Source: CAD feature listing. Evaluate the final solid. Frame: model axes, mm. A direction names the side the tool comes from. Round coordinates to 2 decimals unless told otherwise and drop trailing zeros. Order: outer loops, then holes, each group sorted by start corner. A loop starts at its lowest first (then second) coordinate and runs counter-clockwise, first axis right, second up. Notation, with made-up numbers: M -33,-24.5 L -1,-24.5 A25 cw -1,-8.5 Z; hole C 50,83 d5. An arc over 180 degrees is marked long. Use CSV: the item, a comma, the result in double quotes. Start each with the question number.
```python
from build123d import *

# Parameters (mm, degrees)
F1_DEPTH = 25


with BuildPart() as f1:
    # F0 (on Front) → F1 (new body)
    with BuildSketch(Plane.XZ):
        with BuildLine():
            Line((0, 260), (0, 0))
            Line((0, 0), (2, 0))
            Line((2, 0), (2, 32.289786))
            Line((2, 32.289786), (227.065674, 257.35546))
            Line((227.065674, 257.35546), (268, 257.760407))
            Line((268, 257.760407), (268, 210))
            ThreePointArc((268, 210), (288, 190), (308, 210))
            Line((308, 210), (308, 260))
            Line((308, 260), (306, 260))
            Line((306, 260), (306, 210))
            ThreePointArc((306, 210), (288, 192), (270, 210))
            Line((270, 210), (270, 260))
            Line((270, 260), (0, 260))
        make_face()
        Polygon((2, 35.118214), (2, 255.128978), (224.208987, 257.3272), align=None, mode=Mode.SUBTRACT)
    extrude(amount=F1_DEPTH)


solid = f1.part
```
(1) Section D-D on x = 288. Return loops of the section in (y, z).
(2) Contact query for flat-ended pins moving along their axis: P1, Ø3, axis at x = 110, y = -21.5, coming from the -Z side; P2, Ø7.5, axis at y = -11.5, z = 189, coming from the +X side; P3, Ø5, axis at x = 226, y = -2.5, coming from the -Z side. Output: stop coordinate, or through.
(3) Draft query along Z for faces 1 (the face through (270, -12, 235)), 2 (the face through (137, -12, 260)), 3 (the face through (114.66, -12.32, 147.78)). Return one class per face: pulls with the +Z half, pulls with the -Z half, needs draft (parallel to the pull), parting line crosses it, or undercut.
(4) Section A-A on x = 199.5. Return loops of the section in (y, z), plus the area to 3 significant figures.
(5) Section C-C on y = -21.5. Return loops of the section in (x, z).
(6) Line query: line 1 along X through (y, z) = (-6.75, 213.5); line 2 along X through (y, z) = (-1.5, 241); line 3 along Z through (x, y) = (260.5, -5). Output: solid intervals per line, ascending.
(7) Reachability of faces 4 (the face through (306, -12, 235)), 5 (the face through (2, -12, 16)), 6 (the face through (112.96, -12.32, 143.25)), 7 (the face through (2, -12, 144)) from +Z, -Z, +X, -X, +Y, -Y: full face, straight path, thin tool, end or side. Return the list, or none.
(8) Section B-B on z = 42.5. Return loops of the section in (x, y), plus the area to 3 significant figures.
Results below:
1,outline,"M -25,190 L 0,190 L 0,192 L -25,192 Z"
2,P1,"stops at z = 138.79"
2,P2,"stops at x = 298.12"
2,P3,"stops at z = 253.79"
3,face 1,"needs draft"
3,face 2,"pulls with the +Z half"
3,face 3,"undercut"
4,outline,"M -25,229.79 L 0,229.79 L 0,232.62 L -25,232.62 Z; M -25,257.08 L 0,257.08 L 0,260 L -25,260 Z"
4,area,"144 mm2"
5,outline,"M 0,0 L 2,0 L 2,32.29 L 227.07,257.36 L 268,257.76 L 268,210 A20 ccw 308,210 L 308,260 L 306,260 L 306,210 A18 cw 270,210 L 270,260 L 0,260 Z; hole M 2,35.12 L 224.21,257.33 L 2,255.13 Z"
6,line 1,"x = 0 to 2, 180.38 to 183.21, 268 to 270, 306 to 308"
6,line 2,"x = 0 to 2, 207.88 to 210.71, 268 to 270, 306 to 308"
6,line 3,"z = 257.69 to 260"
7,face 4,"+Z, +Y, -Y"
7,face 5,"-Z, +X, +Y, -Y"
7,face 6,"-Z, +Y, -Y"
7,face 7,"+Y, -Y"
8,outline,"M 0,-25 L 2,-25 L 2,0 L 0,0 Z; M 9.38,-25 L 12.21,-25 L 12.21,0 L 9.38,0 Z"
8,area,"121 mm2"
